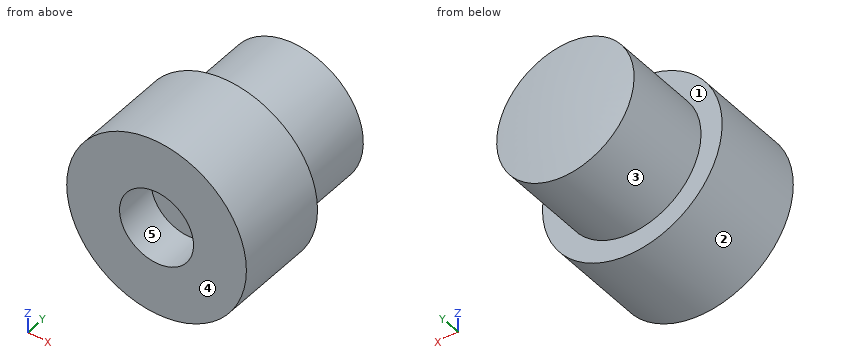
from build123d import *


with BuildPart() as part:
    # Sketch1 → Revolve1 (revolve)
    with BuildSketch(Plane.XY, mode=Mode.PRIVATE) as revolve1_sk:
        with BuildLine():
            Line((-1.75, 0), (-1.75, 2))
            Line((-1.75, 2), (0, 2))
            Line((0, 2), (0, 9))
            ThreePointArc((0, 9), (-1.630426718, 8.933431935), (-3.25, 8.734170872))
            Line((-3.25, 8.734170872), (-3.25, 4.5))
            Line((-3.25, 4.5), (-4.25, 4.5))
            Line((-4.25, 4.5), (-4.25, 0))
            Line((-4.25, 0), (-1.75, 0))
        make_face()
    revolve(revolve1_sk.sketch.rotate(Axis((0, 2, 0), (0, 1, 0)), 270), axis=Axis((0, 2, 0), (0, 1, 0)))


solid = part.part
Part model, mm, in its own coordinate system. Face numbers are marked on the shaded views. A direction names the side the tool comes from. Give positions to 0.01 mm unless a question says otherwise; leave off trailing zeros. Loops run counter-clockwise (first coordinate to the right, second up) from the corner with the lowest first, then second, coordinate; pieces in that order, holes last. Notation, with made-up numbers: (-15.5, 17) -> (31.5, 17) arc R20 cw to (31.5, 31) -> close; hole circle Ø10 at (68.25, 41.25). An arc over 180 degrees is marked (long way). Write each question's results on one line, items separated by ' | '. Start each with the question number.
Q1. Band-saw the part on D-D on y = 4.25. List the corners of the cut face in (x, z), plus the area to 3 significant figures.
Q2. Which spindle directions (+Z, -Z, +X, -X, +Y, -Y) get a long thin tool onto all of the face, cutting with end or side? Do the marked faces 1 and 2. Say none if no direction does.
Q3. Band-saw the part on B-B on x = 0. List the corners of the cut face in (y, z), plus the area to 3 significant figures.
Q4. Wall check: L1, parallel to X at y = 1.15, z = 0; L2, parallel to Y at x = -0.5, z = 3.25; L3, parallel to Z at x = 0.75, y = 1. Give the ranges that are in metal, low to high.
Q5. Pin check, flat tips, straight feed: P1, Ø3, axis at x = 0, z = 0, coming from the -Y side; P2, Ø1, axis at x = -1.5, z = 2, coming from the +Y side; P3, Ø2, axis at y = 7, z = 3.5, coming from the +X side. Stop position of each tip, or through.
Q6. Band-saw the part on C-C on y = 1. List the corners of the cut face in (x, z), plus the area to 3 significant figures.
Q7. Band-saw the part on A-A on z = 0. List the corners of the cut face in (x, y), plus the area to 3 significant figures.
Q8. Pull direction X, two halves, no side cores. Call the marked faces 3, 4 and 5: +X half, -X half, draft (parallel to the pull), parting line (faces both ways), or undercut.
Results are:
1) outline: circle Ø8.5 at (0, 0) | area: 56.7 mm²
2) face 1: +Y | face 2: +Y, -Y
3) outline: (0, -4.25) -> (4.5, -4.25) -> (4.5, -3.25) -> (8.73, -3.25) arc R20 ccw to (8.73, 3.25) -> (4.5, 3.25) -> (4.5, 4.25) -> (0, 4.25) -> (0, 1.75) -> (2, 1.75) -> (2, -1.75) -> (0, -1.75) -> close | area: 59.9 mm²
4) L1: x = -4.25 to -1.75, 1.75 to 4.25 | L2: y = 0 to 4.5 | L3: z = -4.18 to -1.58, 1.58 to 4.18
5) P1: stops at y = 2 | P2: stops at y = 8.9 | P3: stops at x = 2.08
6) outline: circle Ø8.5 at (0, 0); hole circle Ø3.5 at (0, 0) | area: 47.1 mm²
7) outline: (-4.25, 0) -> (-1.75, 0) -> (-1.75, 2) -> (1.75, 2) -> (1.75, 0) -> (4.25, 0) -> (4.25, 4.5) -> (3.25, 4.5) -> (3.25, 8.73) arc R20 ccw to (-3.25, 8.73) -> (-3.25, 4.5) -> (-4.25, 4.5) -> close | area: 59.9 mm²
8) face 3: parting line | face 4: draft | face 5: undercut
